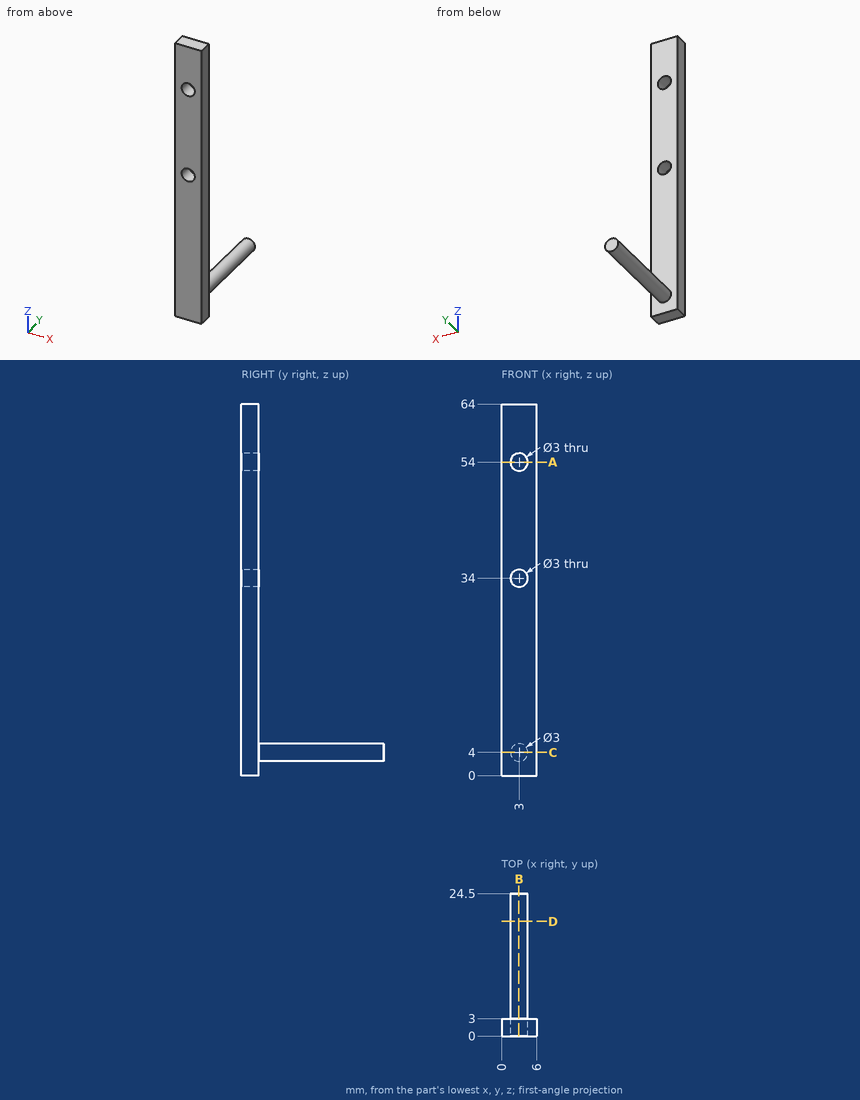
Input: dimensioned drawing with shaded views. Units: mm. Origin: part minimum x, y, z. Round coordinates to 2 decimals unless told otherwise and drop trailing zeros. Order: outer loops, then holes, each group sorted by start corner. A loop starts at its lowest first (then second) coordinate and runs counter-clockwise, first axis right, second up. Notation, with made-up numbers: (75, 30.5) -> (86, 30.5) arc R11 cw to (86, 51.5) -> close; hole circle Ø1 at (31, -29). An arc over 180 degrees is marked (long way). One line per item, written item: value. Start each with the question number.
Q1. Material intervals for probe 1 along Z at (x, y) = (3, 0.75); probe 2 along Y at (x, z) = (2.3, 35.5); probe 3 along Z at (x, y) = (3.2, 19.25), sorted ascending.
Q2. Pin query (flat end, axial travel): pin 1 (1.8 mm diameter, centred on x = 2, z = 38, fed in from +Y); pin 2 (5 mm diameter, centred on y = 20, z = 7, fed in from +X); pin 3 (2 mm diameter, centred on y = 3, z = 25.5, fed in from -X). Return the tip coordinate at first contact, or that it passes through.
Q3. Section query B-B (x = 2.95). Return the cut outline in (y, z).
Q4. Section query D-D (y = 19.75). Return the cut outline in (x, z), plus the area to 3 significant figures.
Q5. Section query C-C (z = 4). Return the cut outline in (x, y), plus the area to 3 significant figures.
Q6. Section query A-A (z = 54). Return the cut outline in (x, y), plus the area to 3 significant figures.
Findings below:
1. probe 1: 0 to 32.5, 35.5 to 52.5, 55.5 to 64
1. probe 2: 0 to 3
1. probe 3: 2.51 to 5.49
2. pin 1: y = 3
2. pin 2: x = 4.41
2. pin 3: x = 0
3. outline: (0, 0) -> (3, 0) -> (3, 2.5) -> (24.5, 2.5) -> (24.5, 5.5) -> (3, 5.5) -> (3, 32.5) -> (0, 32.5) -> close; (0, 35.5) -> (3, 35.5) -> (3, 52.5) -> (0, 52.5) -> close; (0, 55.5) -> (3, 55.5) -> (3, 64) -> (0, 64) -> close
4. outline: circle Ø3 at (3, 4)
4. area: 7.07 mm²
5. outline: (0, 0) -> (6, 0) -> (6, 3) -> (4.5, 3) -> (4.5, 24.5) -> (1.5, 24.5) -> (1.5, 3) -> (0, 3) -> close
5. area: 82.5 mm²
6. outline: (0, 0) -> (1.5, 0) -> (1.5, 3) -> (0, 3) -> close; (4.5, 0) -> (6, 0) -> (6, 3) -> (4.5, 3) -> close
6. area: 9.00 mm²
